from build123d import *

# Parameters (mm, degrees)
SKETCH1_W                 = 20.9
SKETCH1_H                 = 20.9
SKETCH1_W_2               = 12.9
SKETCH1_H_2               = 12.9
BOSS_EXTRUDE1_DEPTH       = 12.7
BOSS_EXTRUDE2_DEPTH       = 3
CUT_EXTRUDE1_DEPTH        = 4
LPATTERN1_COUNT           = 2
LPATTERN1_PITCH           = 13
LPATTERN1_COL_COUNT       = 2
LPATTERN1_COL_PITCH       = 13
CIRPATTERN1_COUNT         = 6
CIRPATTERN1_COPY_1_DEPTH  = 4
CIRPATTERN1_COPY_2_DEPTH  = 4
CIRPATTERN1_COPY_3_DEPTH  = 4
CIRPATTERN1_COPY_4_DEPTH  = 4
CIRPATTERN1_COPY_5_DEPTH  = 4
CIRPATTERN1_COPY_6_DEPTH  = 4
CIRPATTERN1_COPY_7_DEPTH  = 4
CIRPATTERN1_COPY_8_DEPTH  = 4
CIRPATTERN1_COPY_9_DEPTH  = 4
CIRPATTERN1_COPY_10_DEPTH = 4
FILLET1_R                 = 3
FILLET2_R                 = 10
FILLET3_R                 = 2
CHAMFER1_SIZE             = 3


with BuildPart() as part:
    # Sketch1 → Boss-Extrude1 (new body)
    with BuildSketch(Plane(origin=(0, 0, 0), x_dir=(1, 0, 0), z_dir=(0, 1, 0))):
        Rectangle(SKETCH1_W, SKETCH1_H)
        Rectangle(SKETCH1_W_2, SKETCH1_H_2, mode=Mode.SUBTRACT)
    extrude(amount=-BOSS_EXTRUDE1_DEPTH)

    # Sketch2 → Boss-Extrude2 (add)
    with BuildSketch(Plane.XZ.offset(12.7)):
        Polygon((57.735026919, 0), (28.867513459, 50), (-28.867513459, 50), (-57.735026919, 0), (-28.867513459, -50), (28.867513459, -50), align=None)
    extrude(amount=BOSS_EXTRUDE2_DEPTH)

    # Sketch3 → Cut-Extrude1 (cut, through all)
    with BuildSketch(Plane(origin=(0, -12.7, 0), x_dir=(1, 0, 0), z_dir=(0, 1, 0))):
        with BuildLine():
            Line((-34.873066959, 23.598076211), (-18.226787136, 13.987342075))
            ThreePointArc((-18.226787136, 13.987342075), (-17.128710925, 9.889265863), (-21.226787136, 8.791189652))
            Line((-21.226787136, 8.791189652), (-37.873066959, 18.401923789))
            ThreePointArc((-37.873066959, 18.401923789), (-38.97114317, 22.5), (-34.873066959, 23.598076211))
        make_face()
    cut_extrude1 = extrude(amount=-CUT_EXTRUDE1_DEPTH, mode=Mode.SUBTRACT)

    # LPattern1: Cut-Extrude1 ×2
    with Locations(*[Vector(-0.5, 0, 0.866025404) * (i * LPATTERN1_PITCH) for i in range(1, LPATTERN1_COUNT)]):
        add(cut_extrude1, mode=Mode.SUBTRACT)

    # LPattern1 col: Cut-Extrude1 ×2
    with Locations(*[Vector(0.5, 0, -0.866025404) * (i * LPATTERN1_COL_PITCH) for i in range(1, LPATTERN1_COL_COUNT)]):
        add(cut_extrude1, mode=Mode.SUBTRACT)

    # CirPattern1: Cut-Extrude1 ×6 about axis
    cirpattern1_axis = Axis((0, 0, 0), (0, 1, 0))
    for i in range(1, CIRPATTERN1_COUNT):
        add(cut_extrude1.rotate(cirpattern1_axis, i * 360 / CIRPATTERN1_COUNT), mode=Mode.SUBTRACT)

    # CirPattern1 copy 1 sketch → CirPattern1 copy 1 (cut, through all)
    with BuildSketch(Plane(origin=(6.5, -12.7, 11.258330249), x_dir=(0.5, 0, -0.866025404), z_dir=(0, 1, 0))):
        with BuildLine():
            Line((-34.873066959, 23.598076211), (-18.226787136, 13.987342075))
            ThreePointArc((-18.226787136, 13.987342075), (-17.128710925, 9.889265863), (-21.226787136, 8.791189652))
            Line((-21.226787136, 8.791189652), (-37.873066959, 18.401923789))
            ThreePointArc((-37.873066959, 18.401923789), (-38.97114317, 22.5), (-34.873066959, 23.598076211))
        make_face()
    extrude(amount=-CIRPATTERN1_COPY_1_DEPTH, mode=Mode.SUBTRACT)

    # CirPattern1 copy 2 sketch → CirPattern1 copy 2 (cut, through all)
    with BuildSketch(Plane(origin=(13, -12.7, 0), x_dir=(-0.5, 0, -0.866025404), z_dir=(0, 1, 0))):
        with BuildLine():
            Line((-34.873066959, 23.598076211), (-18.226787136, 13.987342075))
            ThreePointArc((-18.226787136, 13.987342075), (-17.128710925, 9.889265863), (-21.226787136, 8.791189652))
            Line((-21.226787136, 8.791189652), (-37.873066959, 18.401923789))
            ThreePointArc((-37.873066959, 18.401923789), (-38.97114317, 22.5), (-34.873066959, 23.598076211))
        make_face()
    extrude(amount=-CIRPATTERN1_COPY_2_DEPTH, mode=Mode.SUBTRACT)

    # CirPattern1 copy 3 sketch → CirPattern1 copy 3 (cut, through all)
    with BuildSketch(Plane(origin=(6.5, -12.7, -11.258330249), x_dir=(-1, 0, 0), z_dir=(0, 1, 0))):
        with BuildLine():
            Line((-34.873066959, 23.598076211), (-18.226787136, 13.987342075))
            ThreePointArc((-18.226787136, 13.987342075), (-17.128710925, 9.889265863), (-21.226787136, 8.791189652))
            Line((-21.226787136, 8.791189652), (-37.873066959, 18.401923789))
            ThreePointArc((-37.873066959, 18.401923789), (-38.97114317, 22.5), (-34.873066959, 23.598076211))
        make_face()
    extrude(amount=-CIRPATTERN1_COPY_3_DEPTH, mode=Mode.SUBTRACT)

    # CirPattern1 copy 4 sketch → CirPattern1 copy 4 (cut, through all)
    with BuildSketch(Plane(origin=(-6.5, -12.7, -11.258330249), x_dir=(-0.5, 0, 0.866025404), z_dir=(0, 1, 0))):
        with BuildLine():
            Line((-34.873066959, 23.598076211), (-18.226787136, 13.987342075))
            ThreePointArc((-18.226787136, 13.987342075), (-17.128710925, 9.889265863), (-21.226787136, 8.791189652))
            Line((-21.226787136, 8.791189652), (-37.873066959, 18.401923789))
            ThreePointArc((-37.873066959, 18.401923789), (-38.97114317, 22.5), (-34.873066959, 23.598076211))
        make_face()
    extrude(amount=-CIRPATTERN1_COPY_4_DEPTH, mode=Mode.SUBTRACT)

    # CirPattern1 copy 5 sketch → CirPattern1 copy 5 (cut, through all)
    with BuildSketch(Plane(origin=(-13, -12.7, 0), x_dir=(0.5, 0, 0.866025404), z_dir=(0, 1, 0))):
        with BuildLine():
            Line((-34.873066959, 23.598076211), (-18.226787136, 13.987342075))
            ThreePointArc((-18.226787136, 13.987342075), (-17.128710925, 9.889265863), (-21.226787136, 8.791189652))
            Line((-21.226787136, 8.791189652), (-37.873066959, 18.401923789))
            ThreePointArc((-37.873066959, 18.401923789), (-38.97114317, 22.5), (-34.873066959, 23.598076211))
        make_face()
    extrude(amount=-CIRPATTERN1_COPY_5_DEPTH, mode=Mode.SUBTRACT)

    # CirPattern1 copy 6 sketch → CirPattern1 copy 6 (cut, through all)
    with BuildSketch(Plane(origin=(-6.5, -12.7, -11.258330249), x_dir=(0.5, 0, -0.866025404), z_dir=(0, 1, 0))):
        with BuildLine():
            Line((-34.873066959, 23.598076211), (-18.226787136, 13.987342075))
            ThreePointArc((-18.226787136, 13.987342075), (-17.128710925, 9.889265863), (-21.226787136, 8.791189652))
            Line((-21.226787136, 8.791189652), (-37.873066959, 18.401923789))
            ThreePointArc((-37.873066959, 18.401923789), (-38.97114317, 22.5), (-34.873066959, 23.598076211))
        make_face()
    extrude(amount=-CIRPATTERN1_COPY_6_DEPTH, mode=Mode.SUBTRACT)

    # CirPattern1 copy 7 sketch → CirPattern1 copy 7 (cut, through all)
    with BuildSketch(Plane(origin=(-13, -12.7, 0), x_dir=(-0.5, 0, -0.866025404), z_dir=(0, 1, 0))):
        with BuildLine():
            Line((-34.873066959, 23.598076211), (-18.226787136, 13.987342075))
            ThreePointArc((-18.226787136, 13.987342075), (-17.128710925, 9.889265863), (-21.226787136, 8.791189652))
            Line((-21.226787136, 8.791189652), (-37.873066959, 18.401923789))
            ThreePointArc((-37.873066959, 18.401923789), (-38.97114317, 22.5), (-34.873066959, 23.598076211))
        make_face()
    extrude(amount=-CIRPATTERN1_COPY_7_DEPTH, mode=Mode.SUBTRACT)

    # CirPattern1 copy 8 sketch → CirPattern1 copy 8 (cut, through all)
    with BuildSketch(Plane(origin=(-6.5, -12.7, 11.258330249), x_dir=(-1, 0, 0), z_dir=(0, 1, 0))):
        with BuildLine():
            Line((-34.873066959, 23.598076211), (-18.226787136, 13.987342075))
            ThreePointArc((-18.226787136, 13.987342075), (-17.128710925, 9.889265863), (-21.226787136, 8.791189652))
            Line((-21.226787136, 8.791189652), (-37.873066959, 18.401923789))
            ThreePointArc((-37.873066959, 18.401923789), (-38.97114317, 22.5), (-34.873066959, 23.598076211))
        make_face()
    extrude(amount=-CIRPATTERN1_COPY_8_DEPTH, mode=Mode.SUBTRACT)

    # CirPattern1 copy 9 sketch → CirPattern1 copy 9 (cut, through all)
    with BuildSketch(Plane(origin=(6.5, -12.7, 11.258330249), x_dir=(-0.5, 0, 0.866025404), z_dir=(0, 1, 0))):
        with BuildLine():
            Line((-34.873066959, 23.598076211), (-18.226787136, 13.987342075))
            ThreePointArc((-18.226787136, 13.987342075), (-17.128710925, 9.889265863), (-21.226787136, 8.791189652))
            Line((-21.226787136, 8.791189652), (-37.873066959, 18.401923789))
            ThreePointArc((-37.873066959, 18.401923789), (-38.97114317, 22.5), (-34.873066959, 23.598076211))
        make_face()
    extrude(amount=-CIRPATTERN1_COPY_9_DEPTH, mode=Mode.SUBTRACT)

    # CirPattern1 copy 10 sketch → CirPattern1 copy 10 (cut, through all)
    with BuildSketch(Plane(origin=(13, -12.7, 0), x_dir=(0.5, 0, 0.866025404), z_dir=(0, 1, 0))):
        with BuildLine():
            Line((-34.873066959, 23.598076211), (-18.226787136, 13.987342075))
            ThreePointArc((-18.226787136, 13.987342075), (-17.128710925, 9.889265863), (-21.226787136, 8.791189652))
            Line((-21.226787136, 8.791189652), (-37.873066959, 18.401923789))
            ThreePointArc((-37.873066959, 18.401923789), (-38.97114317, 22.5), (-34.873066959, 23.598076211))
        make_face()
    extrude(amount=-CIRPATTERN1_COPY_10_DEPTH, mode=Mode.SUBTRACT)

    # Fillet1
    fillet1_edges = [part.edges().sort_by_distance(p)[0] for p in [
        (-16, -14.2, -27.712812921),
        (-16, -14.2, 27.712812921),
        (16, -14.2, 27.712812921),
        (32, -14.2, 0),
        (16, -14.2, -27.712812921),
        (-32, -14.2, 0),
    ]]
    fillet(fillet1_edges, radius=FILLET1_R)

    # Fillet2
    fillet2_edges = [part.edges().sort_by_distance(p)[0] for p in [
        (28.867513459, -14.2, -50),
        (57.735026919, -14.2, 0),
        (28.867513459, -14.2, 50),
        (-28.867513459, -14.2, 50),
        (-57.735026919, -14.2, 0),
        (-28.867513459, -14.2, -50),
    ]]
    fillet(fillet2_edges, radius=FILLET2_R)

    # Fillet3
    fillet3_edges = [part.edges().sort_by_distance(p)[0] for p in [
        (-10.45, -6.35, -10.45),
        (10.45, -6.35, -10.45),
        (10.45, -6.35, 10.45),
        (-10.45, -6.35, 10.45),
    ]]
    fillet(fillet3_edges, radius=FILLET3_R)

    # Chamfer1
    chamfer1_edges = [part.edges().sort_by_distance(p)[0] for p in [
        (-10.45, -12.7, 0),
        (0, -12.7, 10.45),
        (10.45, -12.7, 0),
        (0, -12.7, -10.45),
        (-9.864213562, -12.7, 9.864213562),
        (9.864213562, -12.7, 9.864213562),
        (9.864213562, -12.7, -9.864213562),
        (-9.864213562, -12.7, -9.864213562),
    ]]
    chamfer(chamfer1_edges, length=CHAMFER1_SIZE)


solid = part.part
Design review of the part built by this model. Coordinates are the model's own, in mm. A direction names the side the tool comes from. Round coordinates to 2 decimals unless told otherwise and drop trailing zeros. Write each loop counter-clockwise with the first axis right and the second up, starting at its lowest first coordinate (ties: lowest second). Pieces come first, ordered by that corner, then holes.
Item 1: Consider section A-A on x = 0. Give the boundary of the cut face in (y, z), and give its area (3 significant figures).
Item 2: Consider section D-D on y = -14.25. Count the separate pieces of the cut face and the enclosed holes in it, and give its area (3 significant figures).
Item 3: For pin 1 Ø3.5 at (y, z) = (-13.5, -29) entering from -X; pin 2 Ø3 at (y, z) = (-14, -25) entering from +X; pin 3 Ø1.5 at (x, z) = (-3, -11.5) entering from +Y; pin 4 Ø8 at (y, z) = (-6, 27.5) entering from -X, all flat-tipped, find the tip position at first contact; note any pin that passes through.
Item 4: For faces 4 (the flat face through (29.433, -14.179, 13.529)), 5 (the flat face through (0, -14, 50)), 6 (the flat face through (0, -6, 6.45)), list the 3-axis set-ups (+Z, -Z, +X, -X, +Y, -Y) from which the entire face can be reached by the end or side of a thin tool; tool diameter is ignored.
Item 5: Wall thickness on L1, parallel to X at y = -1, z = -0.5; L2, parallel to X at y = -13, z = -3: over which ranges is each line inside the solid? List them lowest first.
Item 6: Draft analysis for pull direction X (two halves, no side actions). For faces 1 (the conical face through (-10.65, -10.846, 10.699)), 2 (the flat face through (0, -14, -50)), 3 (the cylindrical face through (38.938, -14.179, -22.557)), state which applies: released by +X, released by -X, zero draft, split by the parting line, or undercut.
Item 7: Consider section C-C on z = 38. Give the boundary of the cut face in (x, y).
Item 8: Consider section B-B on y = -6. Give the boundary of the cut face in (x, z).
Check values:
1. outline: (-15.7, -50) - (-12.7, -50) - (-12.7, -45) - (-15.7, -45) - close; (-15.7, -19.78) - (-12.7, -19.78) - (-12.7, -13.45) - (-9.7, -10.45) - (0, -10.45) - (0, -6.45) - (-12.7, -6.45) - (-12.7, 6.45) - (0, 6.45) - (0, 10.45) - (-9.7, 10.45) - (-12.7, 13.45) - (-12.7, 19.78) - (-15.7, 19.78) - close; (-15.7, 45) - (-12.7, 45) - (-12.7, 50) - (-15.7, 50) - close
1. area: 259 mm2
2. separate pieces: 1
2. enclosed holes: 12
2. area: 6,200 mm2
3. pin 1: stops at x = -42
3. pin 2: stops at x = 44.17
3. pin 3: stops at y = -10
3. pin 4: passes through
4. face 4: +Y, -Y
4. face 5: +Z, +X, -X, +Y, -Y
4. face 6: +Y
5. L1: x = -10.45 to -6.45, 6.45 to 10.45
5. L2: x = -55.73 to -37.2, -25.2 to 25.2, 37.2 to 55.73
6. face 1: released by -X
6. face 2: zero draft
6. face 3: undercut
7. outline: (-35.8, -15.7) - (-16, -15.7) - (-16, -12.7) - (-35.8, -12.7) - close; (-10, -15.7) - (-3, -15.7) - (-3, -12.7) - (-10, -12.7) - close; (3, -15.7) - (10, -15.7) - (10, -12.7) - (3, -12.7) - close; (16, -15.7) - (35.8, -15.7) - (35.8, -12.7) - (16, -12.7) - close
8. outline: (-10.45, -8.45) arc R2 ccw to (-8.45, -10.45) - (8.45, -10.45) arc R2 ccw to (10.45, -8.45) - (10.45, 8.45) arc R2 ccw to (8.45, 10.45) - (-8.45, 10.45) arc R2 ccw to (-10.45, 8.45) - close; hole (-6.45, -6.45) - (6.45, -6.45) - (6.45, 6.45) - (-6.45, 6.45) - close
